Autodesk Inventor part; units mm, degrees
ref_plane "YZ Plane" through (0, 0, 0) normal (1, 0, 0) x (0, 1, 0)
ref_plane "XZ Plane" through (0, 0, 0) normal (0, 1, 0) x (-1, 0, 0)
ref_plane "XY Plane" through (0, 0, 0) normal (0, 0, 1) x (1, 0, 0)
sketch "Sketch1" plane through (0, 0, 0) normal (1, 0, 0) x (0, 1, 0)
  line L0 (25.4, 0) -> (25.4, 19.05)
  line L1 (25.4, 19.05) -> (0, 19.05)
  line L2 (0, 19.05) -> (0, -101.6)
  line L3 (0, -101.6) -> (12.7, -101.6)
  line L4 (12.7, -101.6) -> (12.7, -12.7)
  line L5 (12.7, -12.7) -> (15.24, -12.7)
  line L6 (15.24, -12.7) -> (15.24, 0)
  line L7 (15.24, 0) -> (25.4, 0)
  point P0 (0, 0)
  dimension "d10" = 0.508
  dimension "d0" = 19.05
  dimension "d1" = 25.4
  dimension "d2" = 12.7
  dimension "d3" = 15.24
  dimension "d4" = 120.65
  dimension "d5" = 88.9
revolve "Revolution1" add sketch "Sketch1" angle 360 about axis through (0, 0, 19.05) along (0, 0, -1)
chamfer "Chamfer1" distance 1.524 angle 45 2 edges at (0, -25.4, 19.05) (0, -25.4, 0)
fillet "Fillet1" radius 0.508 3 edges at (0, -15.24, 0) (0, -15.24, -12.7) (0, -12.7, -12.7)
properties part number "Shoulder Screw"
Model file for the job. Use its own axes, mm. A direction names the side the tool comes from. Coordinates: 2 decimals unless noted, no trailing zeros. Write each loop counter-clockwise with the first axis right and the second up, starting at its lowest first coordinate (ties: lowest second). Pieces come first, ordered by that corner, then holes. Notation, with made-up numbers: (89.5, 39.5) - (142.5, 39.5) arc R34 cw to (142.5, 71.5) - close; hole circle Ø5 at (34, -29.75). An arc over 180 degrees is marked (long way). One line per item, written item: value. Start each with the question number.
1. Flat gauge pins, fed straight in: pin 1 (2 mm diameter, centred on x = -0.5, z = -30.5, fed in from +Y); pin 2 (4 mm diameter, centred on x = 12.5, z = -82.5, fed in from +Y); pin 3 (4 mm diameter, centred on x = -8, z = -38.5, fed in from -Y). Where does each tip first touch, or does it go through?
2. Slice it at C-C (z = -31). Write the cut outline in (x, y), plus the area to 3 significant figures.
3. Tool access for faces 1 (the flat face through (0, 0, -101.6)), 2 (the cylindrical face through (14.88, -3.3, -6.27)): list every direction of +Z, -Z, +X, -X, +Y, -Y with a clear straight run to the whole face (end or side of a thin tool).
4. Probe line 1 (Z direction, x = 18, y = -6); line 2 (Z direction, x = -2.5, y = -14); line 3 (Y direction, x = 5, z = 4). List the from-to ranges inside material, lowest first. Write a range as from..to.
5. Slice it at A-A (y = 0). Write the cut outline in (x, z), plus the area to 3 significant figures.
Answers below:
1. pin 1: stops at y = 12.7
1. pin 2: stops at y = 7.14
1. pin 3: stops at y = -11.19
2. outline: circle Ø25.4 at (0, 0)
2. area: 507 mm^2
3. face 1: -Z, +X, -X, +Y, -Y
3. face 2: -Z
4. line 1: z = 0..19.05
4. line 2: z = -12.7..19.05
4. line 3: y = -24.9..24.9
5. outline: (-25.4, 1.52) - (-23.88, 0) - (-15.75, 0) arc R0.51 cw to (-15.24, -0.51) - (-15.24, -12.19) arc R0.51 ccw to (-14.73, -12.7) - (-13.21, -12.7) arc R0.51 cw to (-12.7, -13.21) - (-12.7, -101.6) - (12.7, -101.6) - (12.7, -13.21) arc R0.51 cw to (13.21, -12.7) - (14.73, -12.7) arc R0.51 ccw to (15.24, -12.19) - (15.24, -0.51) arc R0.51 cw to (15.75, 0) - (23.88, 0) - (25.4, 1.52) - (25.4, 17.53) - (23.88, 19.05) - (-23.88, 19.05) - (-25.4, 17.53) - close
5. area: 3,610 mm^2
